CAD build for the part. Positions are in the model's coordinates, mm. A direction names the side the tool comes from. Round coordinates to 2 decimals unless told otherwise and drop trailing zeros. Order: outer loops, then holes, each group sorted by start corner. A loop starts at its lowest first (then second) coordinate and runs counter-clockwise, first axis right, second up. Notation, with made-up numbers: (-31.5, -3) -> (-27.5, -3) arc R18 cw to (-27.5, 25) -> close; hole circle Ø9 at (38.25, 13.25). An arc over 180 degrees is marked (long way). Answer as CSV lines item,"result". Start each with the question number.
from build123d import *

# Parameters (mm, degrees)
SKETCH2_R           = 1.7
BOSS_EXTRUDE2_DEPTH = 3
SKETCH3_W           = 30
SKETCH3_H           = 5
BOSS_EXTRUDE3_DEPTH = 5
SKETCH4_W           = 30
SKETCH4_H           = 5
BOSS_EXTRUDE4_DEPTH = 5
SKETCH5_W           = 30
SKETCH5_H           = 4
BOSS_EXTRUDE5_DEPTH = 25
SKETCH6_W           = 30
SKETCH6_H           = 4
BOSS_EXTRUDE8_DEPTH = 25
SKETCH8_R           = 1.2
CUT_EXTRUDE1_DEPTH  = 25
FILLET5_R           = 3.5
FILLET6_R           = 3.5
FILLET7_R           = 3.5
FILLET8_R           = 3.5


with BuildPart() as part:
    # Sketch2 → Boss-Extrude2 (new body)
    with BuildSketch(Plane(origin=(0, 0, 0), x_dir=(0, 1, 0), z_dir=(0, 0, 1))):
        with BuildLine():
            Line((-31.5, -30), (31.5, -30))
            ThreePointArc((31.5, -30), (33.974873734, -28.974873734), (35, -26.5))
            Line((35, -26.5), (35, 26.5))
            ThreePointArc((35, 26.5), (33.974873734, 28.974873734), (31.5, 30))
            Line((31.5, 30), (-31.5, 30))
            ThreePointArc((-31.5, 30), (-33.974873734, 28.974873734), (-35, 26.5))
            Line((-35, 26.5), (-35, -26.5))
            ThreePointArc((-35, -26.5), (-33.974873734, -28.974873734), (-31.5, -30))
        make_face()
        with Locations(Location((20, -14, 0), (0, 0, 270))):
            Circle(SKETCH2_R, mode=Mode.SUBTRACT)
        with Locations(Location((-20, -14, 0), (0, 0, 270))):
            Circle(SKETCH2_R, mode=Mode.SUBTRACT)
        with Locations(Location((20, 14, 0), (0, 0, 270))):
            Circle(SKETCH2_R, mode=Mode.SUBTRACT)
        with Locations(Location((-20, 14, 0), (0, 0, 270))):
            Circle(SKETCH2_R, mode=Mode.SUBTRACT)
        with Locations(Location((31.5, -26.5, 0), (0, 0, 270))):
            Circle(SKETCH2_R, mode=Mode.SUBTRACT)
        with Locations(Location((-31.5, -26.5, 0), (0, 0, 270))):
            Circle(SKETCH2_R, mode=Mode.SUBTRACT)
        with Locations(Location((31.5, 26.5, 0), (0, 0, 270))):
            Circle(SKETCH2_R, mode=Mode.SUBTRACT)
        with Locations(Location((-31.5, 26.5, 0), (0, 0, 270))):
            Circle(SKETCH2_R, mode=Mode.SUBTRACT)
    extrude(amount=BOSS_EXTRUDE2_DEPTH)

    # Sketch3 → Boss-Extrude3 (add)
    with BuildSketch(Plane.YZ.offset(30)):
        with Locations((0, -2.5)):
            Rectangle(SKETCH3_W, SKETCH3_H)
    extrude(amount=-BOSS_EXTRUDE3_DEPTH)

    # Sketch4 → Boss-Extrude4 (add)
    with BuildSketch(Plane(origin=(-30, 0, 0), x_dir=(0, -1, 0), z_dir=(-1, 0, 0))):
        with Locations((0, -2.5)):
            Rectangle(SKETCH4_W, SKETCH4_H)
    extrude(amount=-BOSS_EXTRUDE4_DEPTH)

    # Sketch5 → Boss-Extrude5 (add)
    with BuildSketch(Plane(origin=(-30, 0, 0), x_dir=(0, -1, 0), z_dir=(-1, 0, 0))):
        with Locations((0, -3)):
            Rectangle(SKETCH5_W, SKETCH5_H)
    extrude(amount=BOSS_EXTRUDE5_DEPTH)

    # Sketch6 → Boss-Extrude8 (add)
    with BuildSketch(Plane.YZ.offset(30)):
        with Locations((0, -3)):
            Rectangle(SKETCH6_W, SKETCH6_H)
    extrude(amount=BOSS_EXTRUDE8_DEPTH)

    # Sketch8 → Cut-Extrude1 (cut)
    with BuildSketch(Plane(origin=(0, 0, -1), x_dir=(0, -1, 0), z_dir=(0, 0, 1))):
        with Locations(Location((-8.8, -46, 0), (0, 0, 90))):
            Circle(SKETCH8_R)
        with Locations(Location((8.8, -46, 0), (0, 0, 90))):
            Circle(SKETCH8_R)
        with Locations(Location((-8.8, 46, 0), (0, 0, 90))):
            Circle(SKETCH8_R)
        with Locations(Location((8.8, 46, 0), (0, 0, 90))):
            Circle(SKETCH8_R)
    extrude(amount=-CUT_EXTRUDE1_DEPTH, mode=Mode.SUBTRACT)

    # Fillet5
    fillet5_edges = [part.edges().sort_by_distance(p)[0] for p in [
        (-55, -15, -3),
    ]]
    fillet(fillet5_edges, radius=FILLET5_R)

    # Fillet6
    fillet6_edges = [part.edges().sort_by_distance(p)[0] for p in [
        (-55, 15, -3),
    ]]
    fillet(fillet6_edges, radius=FILLET6_R)

    # Fillet7
    fillet7_edges = [part.edges().sort_by_distance(p)[0] for p in [
        (55, 15, -3),
    ]]
    fillet(fillet7_edges, radius=FILLET7_R)

    # Fillet8
    fillet8_edges = [part.edges().sort_by_distance(p)[0] for p in [
        (55, -15, -3),
    ]]
    fillet(fillet8_edges, radius=FILLET8_R)


solid = part.part
Item 1: Band-saw the part on D-D, the plane y = -23. Give the cut face in (x, z).
Item 2: Mould opens along X. For faces 4 (the cylindrical face through (28.95, -34, 1.48)), 5 (the flat face through (0, 0, 3)), 6 (the cylindrical face through (47.11, -9.26, -2.97)) say: released by +X, released by -X, zero draft, split by the parting line, or undercut.
Item 3: Band-saw the part on C-C, the plane x = -14. Give the cut face in (y, z), and give its area (3 significant figures).
Item 4: Band-saw the part on B-B, the plane y = -8.8. Give the cut face in (x, z).
Item 5: Tool access for faces 1 (the flat face through (30, 0, 1)), 2 (the flat face through (38, 15, -3)), 3 (the flat face through (-25, 0, -2)): list every direction of +Z, -Z, +X, -X, +Y, -Y with a clear straight run to the whole face (end or side of a thin tool).
Item 6: Probe line 1 (Y direction, x = 26.5, z = 2.1); line 2 (Y direction, x = 14, z = 2.4); line 3 (Z direction, x = 24.5, y = -31). List the from-to ranges inside material, lowest first.
Item 7: Pin check, flat tips, straight feed: pin 1 (4 mm diameter, centred on y = -24, z = 0.5, fed in from +X); pin 2 (18 mm diameter, centred on x = -6, y = -8, fed in from -Z); pin 3 (4 mm diameter, centred on x = 44.5, z = -1.5, fed in from -Y); pin 4 (4 mm diameter, centred on x = -46, y = -8.8, fed in from -Z). Stop position of each tip, or through.
Item 8: Band-saw the part on A-A, the plane x = -46. Give the cut face in (y, z), and give its area (3 significant figures).
Values:
1,outline,"(-30, 0) -> (30, 0) -> (30, 3) -> (-30, 3) -> close"
2,face 4,"released by +X"
2,face 5,"zero draft"
2,face 6,"undercut"
3,outline,"(-35, 0) -> (-21.7, 0) -> (-21.7, 3) -> (-35, 3) -> close; (-18.3, 0) -> (18.3, 0) -> (18.3, 3) -> (-18.3, 3) -> close; (21.7, 0) -> (35, 0) -> (35, 3) -> (21.7, 3) -> close"
3,area,"190 mm²"
4,outline,"(-55, -5) -> (-47.2, -5) -> (-47.2, -1) -> (-55, -1) -> close; (-44.8, -5) -> (-25, -5) -> (-25, 0) -> (25, 0) -> (25, -5) -> (44.8, -5) -> (44.8, -1) -> (30, -1) -> (30, 3) -> (-30, 3) -> (-30, -1) -> (-44.8, -1) -> close; (47.2, -5) -> (55, -5) -> (55, -1) -> (47.2, -1) -> close"
5,face 1,"+Z, +X, +Y, -Y"
5,face 2,"-Z, +X, -X, +Y"
5,face 3,"-Z, +Y, -Y"
6,line 1,"-35 to -33.2, -29.8 to 29.8, 33.2 to 35"
6,line 2,"-35 to -21.7, -18.3 to 18.3, 21.7 to 35"
6,line 3,"0 to 3"
7,pin 1,"x = 30"
7,pin 2,"z = 0"
7,pin 3,"y = -15"
7,pin 4,"z = -5"
8,outline,"(-15, -5) -> (-10, -5) -> (-10, -1) -> (-15, -1) -> close; (-7.6, -5) -> (7.6, -5) -> (7.6, -1) -> (-7.6, -1) -> close; (10, -5) -> (15, -5) -> (15, -1) -> (10, -1) -> close"
8,area,"101 mm²"
